The model under review builds one solid part; all positions refer to its coordinate system, in mm. A direction names the side the tool comes from. Round coordinates to 2 decimals unless told otherwise and drop trailing zeros. Write each loop counter-clockwise with the first axis right and the second up, starting at its lowest first coordinate (ties: lowest second). Pieces come first, ordered by that corner, then holes.
Item 1: To check wall thickness, follow L1, parallel to X at y = 0.25, z = -0.75; L2, parallel to X at y = 2.75, z = 0.25; L3, parallel to Z at x = -27, y = 0. State the ranges of each line that lie inside material, in increasing order.
Item 2: Add section A-A (z = 0). Give the boundary of the cut face in (x, y), plus the area to 3 significant figures.
Item 3: Machinability: for faces 1 (the face through (-14.14, -0.54, -2.44)), 2 (the face through (-2.274, -0.867, -3.905)), 3 (the face through (-1, -1.5, 0)), which of the approach directions +Z, -Z, +X, -X, +Y, -Y give a long, thin tool a straight path to every point of the face, cutting with its end or side? Answer none if there is none.
Item 4: Add section C-C (x = -27.5). Give the boundary of the cut face in (y, z).
Item 5: Clearance check with flat-ended pins moving along their axes: pin 1 Ø2 at (y, z) = (1, -1) entering from +X; pin 2 Ø3 at (x, y) = (-4.5, -2) entering from +Z; pin 3 Ø4 at (x, y) = (-4, 2.5) entering from -Z; pin 4 Ø1.5 at (y, z) = (-2.5, -0.5) entering from -X. State where each tip first meets the part, or that it passes through.
Item 6: Add section B-B (x = -9.5). Give the boundary of the cut face in (y, z), plus the area to 3 significant figures.
Item 7: Draft analysis for pull direction Z (two halves, no side actions). For faces 4 (the face through (-24, -1, 2)), 5 (the face through (-28, 0, -2)), 6 (the face through (-1.183, -0.74, 1.305)), state which applies: +Z half, -Z half, draft (parallel to the pull), parting line (faces both ways), or undercut.
```python
from build123d import *

# Parameters (mm, degrees)
CHAMFER1_SIZE      = 0.5
CUT_EXTRUDE1_DEPTH = 2.4


with BuildPart() as part:
    # Sketch1 → Revolve1 (revolve)
    with BuildSketch(Plane.XY):
        with BuildLine():
            Line((0, 0), (0, 3.5))
            ThreePointArc((0, 3.5), (-0.146446609, 3.853553391), (-0.5, 4))
            Line((-0.5, 4), (-4, 4))
            Line((-4, 4), (-4, 2.5))
            Line((-4, 2.5), (-24, 2.5))
            Line((-24, 2.5), (-24, 2))
            Line((-24, 2), (-32, 2))
            Line((-32, 2), (-32, 0))
            Line((-32, 0), (0, 0))
        make_face()
    revolve(axis=Axis((0, 0, 0), (1, 0, 0)))

    # Chamfer1
    chamfer1_edges = [part.edges().sort_by_distance(p)[0] for p in [
        (-32, -2, 0),
    ]]
    chamfer(chamfer1_edges, length=CHAMFER1_SIZE)

    # Sketch2 → Cut-Extrude1 (cut)
    with BuildSketch(Plane(origin=(0, 0, 0), x_dir=(0, 0, -1), z_dir=(1, 0, 0))):
        Polygon((1.732050808, 0), (0.866025404, 1.5), (-0.866025404, 1.5), (-1.732050808, 0), (-0.866025404, -1.5), (0.866025404, -1.5), align=None)
    extrude(amount=-CUT_EXTRUDE1_DEPTH, mode=Mode.SUBTRACT)


solid = part.part
```
Numbers:
1. L1: x = -32 to -2.4
1. L2: x = -4 to 0
1. L3: z = -2 to 2
2. outline: (-32, -1.5) - (-31.5, -2) - (-24, -2) - (-24, -2.5) - (-4, -2.5) - (-4, -4) - (-0.5, -4) arc R0.5 ccw to (0, -3.5) - (0, -1.5) - (-2.4, -1.5) - (-2.4, 1.5) - (0, 1.5) - (0, 3.5) arc R0.5 ccw to (-0.5, 4) - (-4, 4) - (-4, 2.5) - (-24, 2.5) - (-24, 2) - (-31.5, 2) - (-32, 1.5) - close
2. area: 156 mm2
3. face 1: -X
3. face 2: +X, -X
3. face 3: +X
4. outline: circle Ø4 at (0, 0)
5. pin 1: stops at x = 0
5. pin 2: stops at z = 3.96
5. pin 3: stops at z = -3.97
5. pin 4: stops at x = -31.7
6. outline: circle Ø5 at (0, 0)
6. area: 19.6 mm2
7. face 4: draft
7. face 5: parting line
7. face 6: undercut
